```python
from build123d import *

# Parameters (mm, degrees)
BOSS_EXTRUDE1_DEPTH = 1.5
SKETCH2_W           = 15
SKETCH2_H           = 1.5
BOSS_EXTRUDE2_DEPTH = 28.5
SKETCH3_R           = 1.5
CUT_EXTRUDE1_DEPTH  = 62
FILLET1_R           = 1
CUT_EXTRUDE2_REACH  = 63
SKETCH5_R           = 4
SKETCH6_R           = 1
CUT_EXTRUDE3_DEPTH  = 10


with BuildPart() as part:
    # Sketch1 → Boss-Extrude1 (new body)
    with BuildSketch(Plane.XY):
        Polygon((-7.5, -23.042592662), (-7.5, -30.5), (7.5, -30.5), (7.5, -23.042592662), (7.5, 26.84732779), (7.5, 30.5), (-7.5, 30.5), (-7.5, 26.84732779), align=None)
    extrude(amount=BOSS_EXTRUDE1_DEPTH)

    # Sketch2 → Boss-Extrude2 (add)
    with BuildSketch(Plane.XY.offset(1.5)):
        with Locations((0, 29.75)):
            Rectangle(SKETCH2_W, SKETCH2_H)
        with Locations((0, -29.75)):
            Rectangle(SKETCH2_W, SKETCH2_H)
    extrude(amount=BOSS_EXTRUDE2_DEPTH)

    # Sketch3 → Cut-Extrude1 (cut, through all)
    with BuildSketch(Plane(origin=(0, 30.5, 0), x_dir=(1, 0, 0), z_dir=(0, 1, 0))):
        with Locations((0, -22.5)):
            Circle(SKETCH3_R)
    extrude(amount=-CUT_EXTRUDE1_DEPTH, mode=Mode.SUBTRACT)

    # Fillet1
    fillet1_edges = [part.edges().sort_by_distance(p)[0] for p in [
        (0, -30.5, 0),
        (-7.5, -29.75, 30),
        (7.5, -29.75, 30),
        (7.5, 29.75, 30),
        (-7.5, 29.75, 30),
        (0, 30.5, 0),
    ]]
    fillet(fillet1_edges, radius=FILLET1_R)

    # Sketch5 → Cut-Extrude2 (cut, up to next)
    with BuildSketch(Plane(origin=(0, 30.5, 0), x_dir=(1, 0, 0), z_dir=(0, 1, 0)), mode=Mode.PRIVATE) as cut_extrude2_sk1:
        with Locations((0, -22.5)):
            Circle(SKETCH5_R)
    cut_extrude2_tool1 = extrude(cut_extrude2_sk1.sketch, amount=-CUT_EXTRUDE2_REACH, mode=Mode.PRIVATE) & part.part
    add(cut_extrude2_tool1.solids().sort_by_distance((0, 30.5, 22.5))[0], mode=Mode.SUBTRACT)

    # Sketch6 → Cut-Extrude3 (cut)
    with BuildSketch(Plane.XY.offset(1.5)):
        with Locations((0, -14.75)):
            Circle(SKETCH6_R)
        with Locations((0, 1.762)):
            Circle(SKETCH6_R)
    extrude(amount=-CUT_EXTRUDE3_DEPTH, mode=Mode.SUBTRACT)


solid = part.part
```
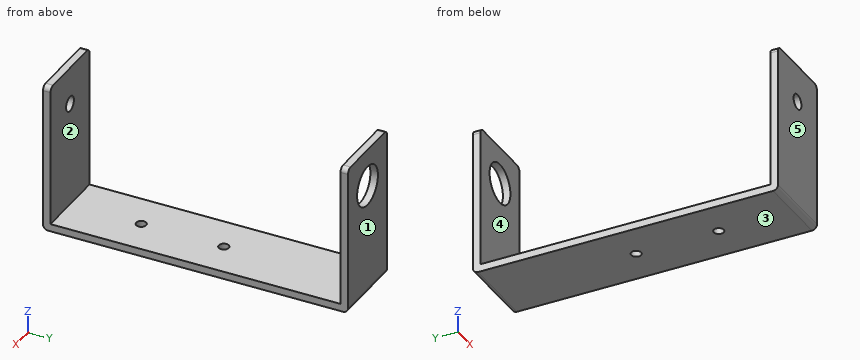
The model under review builds one solid part; all positions refer to its coordinate system, in mm. Face numbers are marked on the shaded views. A direction names the side the tool comes from. Round coordinates to 2 decimals unless told otherwise and drop trailing zeros. Order: outer loops, then holes, each group sorted by start corner. A loop starts at its lowest first (then second) coordinate and runs counter-clockwise, first axis right, second up. Notation, with made-up numbers: (21, 34) -> (70, 34) arc R7 cw to (70, 39) -> close; hole circle Ø3 at (-12, 53.25). An arc over 180 degrees is marked (long way). Use a Markdown table: item, result.
Q1. We need section C-C on z = 22.5. Write out the cut boundary in (x, y).
Values:
| item | result |
|---|---|
| outline | (-7.5, -30.5) -> (-1.5, -30.5) -> (-1.5, -29) -> (-7.5, -29) -> close; (-7.5, 29) -> (-4, 29) -> (-4, 30.5) -> (-7.5, 30.5) -> close; (1.5, -30.5) -> (7.5, -30.5) -> (7.5, -29) -> (1.5, -29) -> close; (4, 29) -> (7.5, 29) -> (7.5, 30.5) -> (4, 30.5) -> close |
Q2. Mouldability with a two-part tool opening along Y and no side actions: class the marked faces 1, 2 and 3 as +Y half, -Y half, draft (parallel to the pull), parting line (faces both ways), or undercut.
Values:
| item | result |
|---|---|
| face 1 | +Y half |
| face 2 | undercut |
| face 3 | draft |
Q3. We need section A-A on y = -14.75. Write out the cut boundary in (x, z), then the cut area to 3 significant figures.
Values:
| item | result |
|---|---|
| outline | (-7.5, 0) -> (-1, 0) -> (-1, 1.5) -> (-7.5, 1.5) -> close; (1, 0) -> (7.5, 0) -> (7.5, 1.5) -> (1, 1.5) -> close |
| area | 19.5 mm^2 |
Q4. We need section B-B on x = 0. Write out the cut boundary in (y, z).
Values:
| item | result |
|---|---|
| outline | (-30.5, 1) arc R1 ccw to (-29.5, 0) -> (-15.75, 0) -> (-15.75, 1.5) -> (-29, 1.5) -> (-29, 21) -> (-30.5, 21) -> close; (-30.5, 24) -> (-29, 24) -> (-29, 30) -> (-30.5, 30) -> close; (-13.75, 0) -> (0.76, 0) -> (0.76, 1.5) -> (-13.75, 1.5) -> close; (2.76, 0) -> (29.5, 0) arc R1 ccw to (30.5, 1) -> (30.5, 18.5) -> (29, 18.5) -> (29, 1.5) -> (2.76, 1.5) -> close; (29, 26.5) -> (30.5, 26.5) -> (30.5, 30) -> (29, 30) -> close |
Q5. Clearance check with flat-ended pins moving along their axes: P1, Ø7.5, axis at x = -0.5, z = 22.5, coming from the +Y side; P2, Ø1.8, axis at x = 0, y = -14.75, coming from the -Z side; P3, Ø4.5, axis at x = 0, y = 5, coming from the +Z side. State where each tip first meets the part, or that it passes through.
Values:
| item | result |
|---|---|
| P1 | stops at y = 30.5 |
| P2 | passes through |
| P3 | stops at z = 1.5 |
Q6. We need section D-D on z = 14.25. Write out the cut boundary in (x, y), then the cut area to 3 significant figures.
Values:
| item | result |
|---|---|
| outline | (-7.5, -30.5) -> (7.5, -30.5) -> (7.5, -29) -> (-7.5, -29) -> close; (-7.5, 29) -> (7.5, 29) -> (7.5, 30.5) -> (-7.5, 30.5) -> close |
| area | 45.0 mm^2 |
Q7. For line 1 (Z direction, x = 0, y = 29.4); line 2 (X direction, y = -29.75, z = 22.5); line 3 (Y direction, x = 0, z = 1.1), list the stretches that pass through material, from the lowest coordinate up.
Values:
| item | result |
|---|---|
| line 1 | z = 0 to 18.5, 26.5 to 30 |
| line 2 | x = -7.5 to -1.5, 1.5 to 7.5 |
| line 3 | y = -30.5 to -15.75, -13.75 to 0.76, 2.76 to 30.5 |
Q8. Tool access review of the marked faces 4 and 5: name each direction out of +Z, -Z, +X, -X, +Y, -Y from which nothing blocks a thin tool from reaching the whole face with its end or side.
Values:
| item | result |
|---|---|
| face 4 | +Z, +X, -X |
| face 5 | +Z, -Z, +X, -X, -Y |
